Geometry check sheet. Reference: the model listing, model coordinates, mm. Give positions to 0.01 mm unless a question says otherwise; leave off trailing zeros. Write each loop counter-clockwise with the first axis right and the second up, starting at its lowest first coordinate (ties: lowest second). Pieces come first, ordered by that corner, then holes. Notation, with made-up numbers: (85.25, 2) -> (90.25, 2) arc R22 cw to (90.25, 15) -> close; hole circle Ø8 at (16.5, -3.5). An arc over 180 degrees is marked (long way). One line per item, written item: value.
from build123d import *

# Parameters (mm, degrees)
F3_DEPTH = 20.001
F4_R     = 10
F5_DEPTH = 20.0010001


with BuildPart() as f1:
    # F0 (on Front) → F1 (revolve)
    with BuildSketch(Plane.XZ):
        Polygon((-4, 0), (-4, 20), (-24.2264973081, 20), (-35.7735026919, 0), align=None)
    revolve(axis=Axis((0, 0, 10), (0, 0, 1)))

    # F2 (on Top) → F3 (cut, through all)
    with BuildSketch(Plane.XY):
        with BuildLine():
            ThreePointArc((-17.2168920075, 31.3579674795), (0, 24.2264973081), (17.2168920075, 31.3579674795))
            ThreePointArc((17.2168920075, 31.3579674795), (0, 35.7735026919), (-17.2168920075, 31.3579674795))
        make_face()
        with BuildLine():
            ThreePointArc((31.3579674795, -17.2168920075), (34.6520405524, -8.887045651), (35.7735026919, 0))
            ThreePointArc((35.7735026919, 0), (34.6520405524, 8.887045651), (31.3579674795, 17.2168920075))
            ThreePointArc((31.3579674795, 17.2168920075), (24.2264973081, 0), (31.3579674795, -17.2168920075))
        make_face()
        with BuildLine():
            ThreePointArc((-17.2168920075, -31.3579674795), (0, -35.7735026919), (17.2168920075, -31.3579674795))
            ThreePointArc((17.2168920075, -31.3579674795), (0, -24.2264973081), (-17.2168920075, -31.3579674795))
        make_face()
        with BuildLine():
            ThreePointArc((-31.3579674795, -17.2168920075), (-24.2264973081, 0), (-31.3579674795, 17.2168920075))
            ThreePointArc((-31.3579674795, 17.2168920075), (-35.7735026919, 0), (-31.3579674795, -17.2168920075))
        make_face()
    extrude(amount=F3_DEPTH, mode=Mode.SUBTRACT)

    # F4 (on Top) → F5 (cut, through all)
    with BuildSketch(Plane.XY):
        with Locations((-12.6478431701, -12.6478431701)):
            Circle(F4_R)
        with Locations((12.6478431701, -12.6478431701)):
            Circle(F4_R)
        with Locations((12.6478431701, 12.6478431701)):
            Circle(F4_R)
        with Locations((-12.6478431701, 12.6478431701)):
            Circle(F4_R)
    extrude(amount=F5_DEPTH, mode=Mode.SUBTRACT)


solid = f1.part
1) Depth check by flat-ended pin: pin 1 Ø12 at (x, y) = (-12.65, -12.65) entering from +Z; pin 2 Ø8 at (y, z) = (-21, 10.5) entering from -X; pin 3 Ø2 at (y, z) = (-8, 17) entering from +X; pin 4 Ø12 at (x, y) = (24, 2.5) entering from -Z. Enter the tip coordinate at first touch or a pass-through.
Verdict:
pin 1: through
pin 2: x = -25.54
pin 3: x = 25.37
pin 4: z = 0
2) Sectioned sample at B-B on z = 5.5. Record the cut outline in (x, y), plus the area to 3 significant figures.
Verdict:
outline: (-29.12, -14.64) arc R32.6 ccw to (-14.64, -29.12) arc R24.35 cw to (14.64, -29.12) arc R32.6 ccw to (29.12, -14.64) arc R24.35 cw to (29.12, 14.64) arc R32.6 ccw to (14.64, 29.12) arc R24.35 cw to (-14.64, 29.12) arc R32.6 ccw to (-29.12, 14.64) arc R24.35 cw to start; hole circle Ø20 at (-12.65, -12.65); hole circle Ø20 at (-12.65, 12.65); hole circle Ø8 at (0, 0); hole circle Ø20 at (12.65, -12.65); hole circle Ø20 at (12.65, 12.65)
area: 1,370 mm^2
3) Sectioned sample at A-A on z = 13.75. Record the cut outline in (x, y).
Verdict:
outline: (-26.16, -9.51) arc R27.83 ccw to (-20.56, -18.77) arc R10 cw (long way) to (-18.77, -20.56) arc R27.83 ccw to (-9.51, -26.16) arc R24.35 cw to (9.51, -26.16) arc R27.83 ccw to (18.77, -20.56) arc R10 cw (long way) to (20.56, -18.77) arc R27.83 ccw to (26.16, -9.51) arc R24.35 cw to (26.16, 9.51) arc R27.83 ccw to (20.56, 18.77) arc R10 cw (long way) to (18.77, 20.56) arc R27.83 ccw to (9.51, 26.16) arc R24.35 cw to (-9.51, 26.16) arc R27.83 ccw to (-18.77, 20.56) arc R10 cw (long way) to (-20.56, 18.77) arc R27.83 ccw to (-26.16, 9.51) arc R24.35 cw to start; hole circle Ø8 at (0, 0)
4) Scan lines: probe 1 along X at (y, z) = (0, 5); probe 2 along X at (y, z) = (11, 7.75); probe 3 along Y at (x, z) = (8, 3). Record each from-to range of solid material in increasing order.
Verdict:
probe 1: -24.23 to -4, 4 to 24.23
probe 2: -26.85 to -22.51, -2.78 to 2.78, 22.51 to 26.85
probe 3: -25.58 to -21.5, -3.79 to 3.79, 21.5 to 25.58
5) Mould release check, pull along Y, two halves, no side actions. Record for faces 1 (the conical face through (21.5, 21.04, 9.86)), 2 (the flat face through (-4, 2, 20)), 3 (the conical face through (21.04, -21.5, 9.86)), 4 (the cylindrical face through (-8.03, 3.78, 9.86)): released by +Y, released by -Y, zero draft, split by the parting line, or undercut.
Verdict:
face 1: released by +Y
face 2: zero draft
face 3: released by -Y
face 4: undercut
6) Sectioned sample at C-C on y = 19.5. Give the number of separate pieces and of enclosed holes in the cut face, plus the area to 3 significant figures.
Verdict:
separate pieces: 3
enclosed holes: 0
area: 356 mm^2
